Check sheet for the modelled part. Datum: model origin and axes. Units: mm. Round coordinates to 2 decimals unless told otherwise and drop trailing zeros. Order: outer loops, then holes, each group sorted by start corner. A loop starts at its lowest first (then second) coordinate and runs counter-clockwise, first axis right, second up. Notation, with made-up numbers: (-27, -10.75) -> (14, -10.75) arc R31 cw to (14, 17.25) -> close; hole circle Ø4 at (-20, 33). An arc over 180 degrees is marked (long way). Answer as CSV lines item,"result". Start each with the question number.
from build123d import *

# Parameters (mm, degrees)
F0_W           = 69.85
F0_H           = 44.45
F1_DEPTH       = 4.826
F2_D           = 6.35
F2_CSINK_D     = 11.43
F2_CSINK_ANGLE = 82


with BuildPart() as f1:
    # F0 (on Front) → F1 (new body)
    with BuildSketch(Plane.XZ):
        with Locations((-0.127, 0)):
            Rectangle(F0_W, F0_H)
    extrude(amount=F1_DEPTH)

    # F2 (through all)
    with Locations(Plane(origin=(0, 0, 0), x_dir=(1, 0, 0), z_dir=(0, 1, 0))):
        with Locations((-19.05, -3.937), (18.796, -3.937)):
            CounterSinkHole(F2_D / 2, F2_CSINK_D / 2, counter_sink_angle=F2_CSINK_ANGLE)


solid = f1.part
1) Section check A-A on x = -19.05. Record the cut outline in (y, z) (3 decimals).
2) Section check B-B on y = -3.8. Record the cut outline in (x, z) (3 decimals).
3) Mould release check, pull along Z, two halves, no side actions. Record for faces 1 (the face through (-1, -4.826, 0)), 2 (the face through (-22.2, -2.78, 2.95)), 3 (the face through (-1, -2, -22.225)): released by +Z, released by -Z, zero draft, split by the parting line, or undercut.
4) Material ranges on line 1 along Z through (x, y) = (-19.05, -4.4) (3 decimals); line 2 along X through (y, z) = (-0.75, 2); line 3 along X through (y, z) = (-1.65, 1), recorded low to high.
5) Depth check by flat-ended pin: pin 1 Ø8.5 at (x, z) = (18.796, 3.937) entering from +Y. Enter the tip coordinate at first touch or a pass-through.
Solutions:
1,outline,"(-4.826, -22.225) -> (0, -22.225) -> (0, -1.778) -> (-2.922, 0.762) -> (-4.826, 0.762) -> close; (-4.826, 7.112) -> (-2.922, 7.112) -> (0, 9.652) -> (0, 22.225) -> (-4.826, 22.225) -> close"
2,outline,"(-35.052, -22.225) -> (34.798, -22.225) -> (34.798, 22.225) -> (-35.052, 22.225) -> close; hole circle Ø6.35 at (-19.05, 3.937); hole circle Ø6.35 at (18.796, 3.937)"
3,face 1,"zero draft"
3,face 2,"undercut"
3,face 3,"released by -Z"
4,line 1,"z = -22.225 to 0.762, 7.112 to 22.225"
4,line 2,"x = -35.05 to -23.73, -14.37 to 14.12, 23.47 to 34.8"
4,line 3,"x = -35.05 to -22.16, -15.94 to 15.68, 21.91 to 34.8"
5,pin 1,"stops at y = -1.69"
